Input: part model. Units: mm. Frame: model coordinates. A direction names the side the tool comes from. Coordinates: 2 decimals unless noted, no trailing zeros. Write each loop counter-clockwise with the first axis right and the second up, starting at its lowest first coordinate (ties: lowest second). Pieces come first, ordered by that corner, then holes. Notation, with made-up numbers: (-22, 54.5) - (-5, 54.5) arc R26 cw to (-5, 70.5) - close; hole circle Ø4 at (85, -23.75). An arc over 180 degrees is marked (long way). Use CSV: the item, a comma, the result in double quotes.
```python
from build123d import *

# Parameters (mm, degrees)
EXTRUDE_1_DEPTH             = 2697
SKETCH_2_W                  = 61
SKETCH_2_H                  = 134
EXTRUDE_2_DEPTH             = 6
SKETCH_3_W                  = 61
SKETCH_3_H                  = 134
EXTRUDE_3_DEPTH             = 6
HOLE_WIZARD_16_0_16_1_D     = 16
HOLE_WIZARD_16_0_16_1_DEPTH = 5
HOLE_WIZARD_16_0_16_1_TIP   = 4.806884952
HOLE_WIZARD_16_0_16_2_D     = 16
PATTERN_LINEAR_1_COUNT      = 2
PATTERN_LINEAR_1_PITCH      = 50
HOLE_WIZARD_16_0_16_3_D     = 16
HOLE_WIZARD_16_0_16_4_D     = 16
PATTERN_LINEAR_2_COUNT      = 2
PATTERN_LINEAR_2_PITCH      = 50


with BuildPart() as part:
    # Model → 凸台-拉伸1 (new body)
    with BuildSketch(Plane.XY):
        with BuildLine():
            Line((11739.240027423, -58278.413223948), (11736.240027423, -58275.413223948))
            Line((11736.240027423, -58275.413223948), (11691.240027423, -58275.413223948))
            Line((11691.240027423, -58275.413223948), (11688.240027423, -58278.413223948))
            Line((11688.240027423, -58278.413223948), (11681.240027423, -58278.413223948))
            Line((11681.240027423, -58278.413223948), (11681.240027423, -58270.413223948))
            Line((11681.240027423, -58270.413223948), (11739.240027423, -58270.413223948))
            ThreePointArc((11739.240027423, -58270.413223948), (11741.361347766, -58269.534544291), (11742.240027423, -58267.413223948))
            Line((11742.240027423, -58267.413223948), (11742.240027423, -58139.413223948))
            ThreePointArc((11742.240027423, -58139.413223948), (11741.361347766, -58137.291903604), (11739.240027423, -58136.413223948))
            Line((11739.240027423, -58136.413223948), (11681.240027423, -58136.413223948))
            Line((11681.240027423, -58136.413223948), (11681.240027423, -58128.413223948))
            Line((11681.240027423, -58128.413223948), (11688.240027423, -58128.413223948))
            Line((11688.240027423, -58128.413223948), (11691.240027423, -58131.413223948))
            Line((11691.240027423, -58131.413223948), (11736.240027423, -58131.413223948))
            Line((11736.240027423, -58131.413223948), (11739.240027423, -58128.413223948))
            Line((11739.240027423, -58128.413223948), (11746.240027423, -58128.413223948))
            Line((11746.240027423, -58128.413223948), (11746.240027423, -58278.413223948))
            Line((11746.240027423, -58278.413223948), (11739.240027423, -58278.413223948))
        make_face()
    extrude(amount=EXTRUDE_1_DEPTH)

    # 草图2 → 凸台-拉伸2 (add)
    with BuildSketch(Plane.XY.offset(2697)):
        with Locations((11711.740027423, -58203.413223948)):
            Rectangle(SKETCH_2_W, SKETCH_2_H)
    extrude(amount=-EXTRUDE_2_DEPTH)

    # 草图3 → 凸台-拉伸3 (add)
    with BuildSketch(Plane(origin=(0, 0, 0), x_dir=(-1, 0, 0), z_dir=(0, 0, -1))):
        with Locations((-11711.740027423, -58203.413223948)):
            Rectangle(SKETCH_3_W, SKETCH_3_H)
    extrude(amount=-EXTRUDE_3_DEPTH)

    # Ø16.0 (16) 直径孔1
    with Locations(Plane.ZY.offset(-11742.240027423)):
        with Locations((200, -58208.413223948), (800, -58208.413223948), (1400, -58208.413223948), (2000, -58208.413223948), (2600, -58208.413223948)):
            Hole(HOLE_WIZARD_16_0_16_1_D / 2, depth=HOLE_WIZARD_16_0_16_1_DEPTH)
            with Locations((0, 0, -(HOLE_WIZARD_16_0_16_1_DEPTH + HOLE_WIZARD_16_0_16_1_TIP / 2))):  # 118° drill point
                Cone(0, HOLE_WIZARD_16_0_16_1_D / 2, HOLE_WIZARD_16_0_16_1_TIP, mode=Mode.SUBTRACT)

    # Ø16.0 (16) 直径孔2 (through all)
    with Locations(Plane(origin=(0, -58275.413223948, 0), x_dir=(-1, 0, 0), z_dir=(0, -1, 0))):
        with Locations((-11713.740027423, -2647)):
            hole_wizard_16_0_16_2 = Hole(HOLE_WIZARD_16_0_16_2_D / 2)

    # 阵列(线性)1: Ø16.0 (16) 直径孔2 ×2
    with Locations(*[(0, 0, -i * PATTERN_LINEAR_1_PITCH) for i in range(1, PATTERN_LINEAR_1_COUNT)]):
        add(hole_wizard_16_0_16_2, mode=Mode.SUBTRACT)

    # Ø16.0 (16) 直径孔3 (through all)
    with Locations(Plane(origin=(0, -58275.413223948, 0), x_dir=(-1, 0, 0), z_dir=(0, -1, 0))):
        with Locations((-11713.740027423, -47), (-11713.740027423, -97)):
            Hole(HOLE_WIZARD_16_0_16_3_D / 2)

    # Ø16.0 (16) 直径孔4 (through all)
    with Locations(Plane.XY.offset(2697)):
        with Locations((11713.740027423, -58178.413223948)):
            hole_wizard_16_0_16_4 = Hole(HOLE_WIZARD_16_0_16_4_D / 2)

    # 阵列(线性)2: Ø16.0 (16) 直径孔4 ×2
    with Locations(*[(0, -i * PATTERN_LINEAR_2_PITCH, 0) for i in range(1, PATTERN_LINEAR_2_COUNT)]):
        add(hole_wizard_16_0_16_4, mode=Mode.SUBTRACT)


solid = part.part
```
(1) Draft query along Y for faces 4 (the flat face through (11742.24, -58204, 1330)), 5 (the flat face through (11714, -58202, 0)), 6 (the flat face through (11713, -58131.413, 1330)). Return one class per face: pulls with the +Y half, pulls with the -Y half, needs draft (parallel to the pull), parting line crosses it, or undercut.
Check values:
face 4,"undercut"
face 5,"needs draft"
face 6,"pulls with the +Y half"
(2) Ray query, probe 1 along Z at (x, y) = (11710, -58236); probe 2 along Y at (x, z) = (11708, 1512.5); probe 3 along Y at (x, z) = (11691, 1613.5). Return the intervals inside material, ascending. Write a range as from..to.
Check values:
probe 1,"0..6, 2691..2697"
probe 2,"-58275.41..-58270.41, -58136.41..-58131.41"
probe 3,"-58275.65..-58270.41, -58136.41..-58131.17"
(3) Pin query (flat end, axial travel): pin 1 Ø6 at (x, z) = (11693, 543.5) entering from -Y; pin 2 Ø21 at (x, y) = (11713.74, -58178.41) entering from +Z; pin 3 Ø12 at (x, z) = (11714.5, 1905.5) entering from -Y; pin 4 Ø1.5 at (x, z) = (11734.5, 1976) entering from +Y. Return the tip coordinate at first contact, or that it passes through.
Check values:
pin 1,"y = -58276.65"
pin 2,"z = 2697"
pin 3,"y = -58275.41"
pin 4,"y = -58131.41"
(4) Cut plane A-A on z = 1131. Return loops of the section in (x, y).
Check values:
outline,"(11681.24, -58278.41) - (11688.24, -58278.41) - (11691.24, -58275.41) - (11736.24, -58275.41) - (11739.24, -58278.41) - (11746.24, -58278.41) - (11746.24, -58128.41) - (11739.24, -58128.41) - (11736.24, -58131.41) - (11691.24, -58131.41) - (11688.24, -58128.41) - (11681.24, -58128.41) - (11681.24, -58136.41) - (11739.24, -58136.41) arc R3 cw to (11742.24, -58139.41) - (11742.24, -58267.41) arc R3 cw to (11739.24, -58270.41) - (11681.24, -58270.41) - close"
(5) Reachability of faces 1 (the flat face through (11681.24, -58276, 1355)), 2 (the flat face through (11710, -58270.413, 1330)), 3 (the flat face through (11714, -58275.413, 1330)) from +Z, -Z, +X, -X, +Y, -Y: full face, straight path, thin tool, end or side. Return the list, or none.
Check values:
face 1,"+Z, -Z, -X, +Y, -Y"
face 2,"-X"
face 3,"+Z, -Z, -Y"
